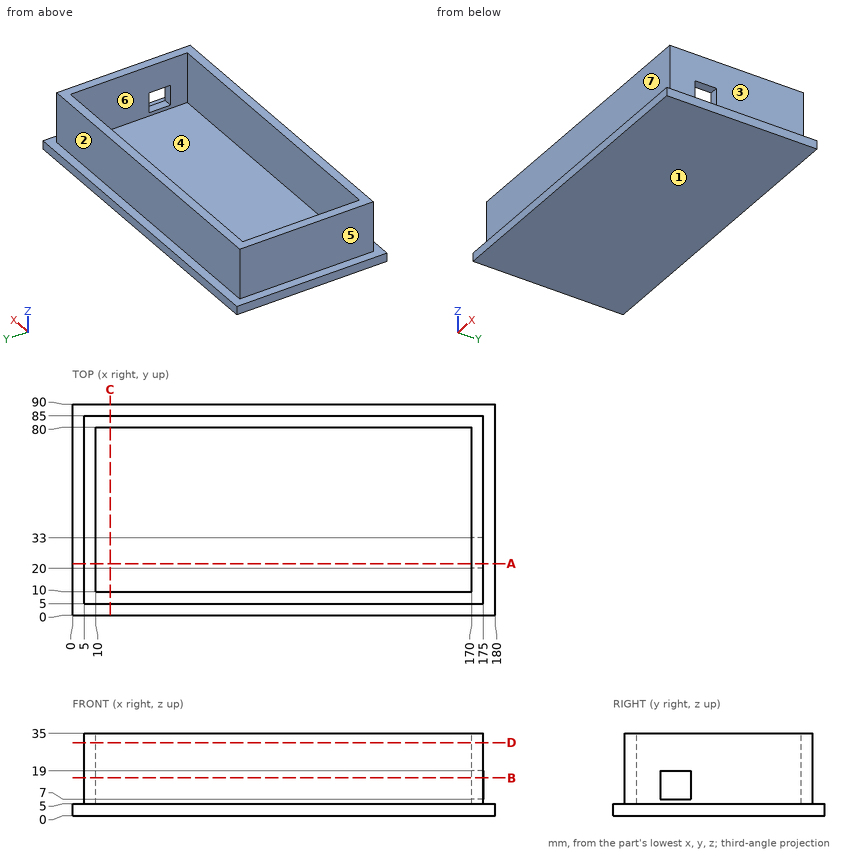
Part print with two shaded views. Sizes in mm from the minimum x, y, z corner. A direction names the side the tool comes from. Coordinates: 2 decimals unless noted, no trailing zeros. Write each loop counter-clockwise with the first axis right and the second up, starting at its lowest first coordinate (ties: lowest second). Pieces come first, ordered by that corner, then holes. Notation, with made-up numbers: M 83.5,67 L 130.5,67 A15 ccw 130.5,80 Z; hole C 64.5,-11 d6. An arc over 180 degrees is marked long. Return JSON: item names as keys, results as strings.
Item 1: Two-plate mould, pull along X, no slides. Class the marked faces 5, 6 and 7: +X half, -X half, draft (parallel to the pull), parting line (faces both ways), or undercut.
Findings below:
{"face 5": "-X half", "face 6": "undercut", "face 7": "draft"}
Item 2: Slice it at C-C, the plane x = 16. Write the cut outline in (y, z), and give its area (3 significant figures).
Findings below:
{"outline": "M 0,0 L 90,0 L 90,5 L 85,5 L 85,35 L 80,35 L 80,5 L 10,5 L 10,35 L 5,35 L 5,5 L 0,5 Z", "area": "750 mm2"}
Item 3: Slice it at B-B, the plane z = 16. Write the cut outline in (x, y).
Findings below:
{"outline": "M 5,5 L 175,5 L 175,20 L 170,20 L 170,10 L 10,10 L 10,80 L 170,80 L 170,33 L 175,33 L 175,85 L 5,85 Z"}
Item 4: Which spindle directions (+Z, -Z, +X, -X, +Y, -Y) get a long thin tool onto all of the face, cutting with end or side? Do the marked faces 1, 2, 3 and 4. Say none if no direction does.
Findings below:
{"face 1": "-Z, +X, -X, +Y, -Y", "face 2": "+Z, +X, -X, +Y", "face 3": "+Z, +X, +Y, -Y", "face 4": "+Z"}
Item 5: Drop flat-ended pins along their axis: pin 1 Ø15 at (x, z) = (82.5, 25.5) entering from -Y; pin 2 Ø4 at (x, z) = (55.5, 15.5) entering from +Y; pin 3 Ø1.5 at (x, y) = (101, 58) entering from -Z; pin 4 Ø9 at (y, z) = (56, 18) entering from -X. Give the stop position or say it passes through.
Findings below:
{"pin 1": "stops at y = 5", "pin 2": "stops at y = 85", "pin 3": "stops at z = 0", "pin 4": "stops at x = 5"}
Item 6: Probe line 1 (X direction, y = 77.5, z = 23); line 2 (Y direction, x = 56, z = 10); line 3 (Z direction, x = 96, y = 16.5). List the from-to ranges inside material, lowest first. Write a range as from..to.
Findings below:
{"line 1": "x = 5..10, 170..175", "line 2": "y = 5..10, 80..85", "line 3": "z = 0..5"}
Item 7: Slice it at D-D, the plane z = 31. Write the cut outline in (x, y), and give its area (3 significant figures).
Findings below:
{"outline": "M 5,5 L 175,5 L 175,85 L 5,85 Z; hole M 10,10 L 170,10 L 170,80 L 10,80 Z", "area": "2,400 mm2"}
Item 8: Slice it at A-A, the plane y = 22. Write the cut outline in (x, z), and give its area (3 significant figures).
Findings below:
{"outline": "M 0,0 L 180,0 L 180,5 L 175,5 L 175,7 L 170,7 L 170,5 L 10,5 L 10,35 L 5,35 L 5,5 L 0,5 Z; M 170,19 L 175,19 L 175,35 L 170,35 Z", "area": "1,140 mm2"}
